Model file for the job. Use its own axes, mm. A direction names the side the tool comes from. Round coordinates to 2 decimals unless told otherwise and drop trailing zeros. Order: outer loops, then holes, each group sorted by start corner. A loop starts at its lowest first (then second) coordinate and runs counter-clockwise, first axis right, second up. Notation, with made-up numbers: (24, 19) - (29, 19) arc R28 cw to (29, 58) - close; hole circle Ø5 at (40.25, -17). An arc over 180 degrees is marked (long way). Put each result on its own line as item: value. Start each with the question number.
Item 1: Probe probe 1 along Z at (x, y) = (188.5, 18); probe 2 along X at (y, z) = (20, 56); probe 3 along X at (y, z) = (45, 133.5). List the from-to ranges inside material, lowest first.
Item 2: Mould opens along Z. For faces 4 (the face through (104, 0, 74)), 5 (the face through (195, 20, 50)), 6 (the face through (195.5, 15.8, 90)), 7 (the face through (195, 20, 100)) say: pulls with the +Z half, pulls with the -Z half, needs draft (parallel to the pull), parting line crosses it, or undercut.
Item 3: Which spindle directions (+Z, -Z, +X, -X, +Y, -Y) get a long thin tool onto all of the face, cutting with end or side? Do faces 1 (the face through (196, 15, 60)), 2 (the face through (89.36, 41.67, 73.95)), 3 (the face through (196, 40, 95)). Say none if no direction does.
Item 4: Saw through at C-C on x = 66.5. List the corners of the cut face in (y, z).
Item 5: Saw through at B-B on x = 145.5. List the corners of the cut face in (y, z).
Item 6: Saw through at A-A on z = 65.5. List the corners of the cut face in (x, y).
Item 7: Pin check, flat tips, straight feed: pin 1 Ø20 at (x, y) = (197, 11) entering from +Z; pin 2 Ø8 at (x, z) = (189.5, 55) entering from +Y; pin 3 Ø2 at (y, z) = (60, 51) entering from -X; pin 4 Ø17.5 at (x, y) = (206.26, 20) entering from -Z. Stop position of each tip, or through.
Autodesk Inventor part; units mm, degrees
ref_plane "YZ Plane" through (0, 0, 0) normal (1, 0, 0) x (0, 1, 0)
ref_plane "XZ Plane" through (0, 0, 0) normal (0, 1, 0) x (-1, 0, 0)
ref_plane "XY Plane" through (0, 0, 0) normal (0, 0, 1) x (1, 0, 0)
sketch "Sketch1" plane through (0, 0, 0) normal (0, 0, 1) x (1, 0, 0)
  line L0 (0, 0) -> (181.2616, 84.5237)
  line L1 (0, 0) -> (200, 0) construction
  line L2 (0, 0) -> (181.2616, 0)
  line L3 (181.2616, 84.5237) -> (181.2616, 0)
  dimension "d2" = 200
  dimension "d3" = 25
extrude "Extrusion1" add sketch "Sketch1" along normal blind 150
sketch "Sketch2" plane through (0, 0, 150) normal (0, 0, 1) x (1, 0, 0)
  point P0 (0, 0)
sketch "Sketch3" plane through (181.2616, 0, 0) normal (1, 0, 0) x (0, 0, -1)
  line L0 (-100, 0) -> (-50, 0)
  line L1 (-50, 0) -> (-50, 40)
  line L2 (-50, 40) -> (-100, 40)
  line L3 (-100, 40) -> (-100, 0)
  dimension "d10" = 50
  dimension "d11" = 40
extrude "Extrusion2" add sketch "Sketch3" along normal blind 50
sketch "Sketch5" plane through (231.2616, 0, 0) normal (1, 0, 0) x (0, 0, -1)
  point P0 (0, 0)
sketch "Sketch6" plane through (231.2616, 0, 0) normal (1, 0, 0) x (0, 0, -1)
  line L0 (0, 0) -> (60, 0) construction
  line L1 (-60, 40) -> (-90, 40)
  line L2 (-90, 40) -> (-90, 0)
  line L3 (-90, 0) -> (-60, 0)
  line L4 (-60, 0) -> (-60, 40)
  dimension "d27" = 30
  dimension "d28" = 40
extrude "Extrusion3" cut sketch "Sketch6" against normal blind 50
sketch "Sketch8" plane through (181.2616, 0, 100) normal (0, 0, 1) x (1, 0, 0)
  line L0 (50, 0) -> (50, 40)
  line L1 (0, 40) -> (0, 0)
  line L2 (0, 40) -> (50, 40)
  line L3 (0, 0) -> (50, 0)
  point P0 (-181.2616, 0)
  point P1 (25, 20)
hole "Hole2" at (206.2616, 20, 100) direction (0, 0, -1) diameter 22 end through all
fillet "Fillet1" radius 20 1 edges at (231.2616, 40, 95)
fillet "Fillet2" radius 20 1 edges at (231.2616, 0, 95)
fillet "Fillet3" radius 20 1 edges at (231.2616, 40, 55)
fillet "Fillet4" radius 20 1 edges at (231.2616, 0, 55)
properties part number "RoboArm 2020 scoop"
Results found:
1. probe 1: z = 50 to 60, 90 to 100
1. probe 2: x = 42.89 to 195.26, 217.26 to 231.26
1. probe 3: x = 96.5 to 181.26
2. face 4: needs draft
2. face 5: pulls with the -Z half
2. face 6: undercut
2. face 7: pulls with the +Z half
3. face 1: +X, +Y, -Y
3. face 2: +Z, -Z, -X, +Y
3. face 3: +Z, -Z, +X, +Y
4. outline: (0, 0) - (31.01, 0) - (31.01, 150) - (0, 150) - close
5. outline: (0, 0) - (67.85, 0) - (67.85, 150) - (0, 150) - close
6. outline: (0, 0) - (181.26, 0) - (181.26, 84.52) - close
7. pin 1: stops at z = 100
7. pin 2: stops at y = 40
7. pin 3: stops at x = 126.53
7. pin 4: passes through
